```python
from build123d import *

# Parameters (mm, degrees)
SCHIZZO1_W                   = 205
SCHIZZO1_H                   = 100
ESTRUSIONE_ESTRUSIONE1_DEPTH = 20
SCHIZZO2_W                   = 20
SCHIZZO2_H                   = 100
ESTRUSIONE_ESTRUSIONE2_DEPTH = 65
TAGLIO_ESTRUSIONE1_DEPTH     = 20
SCHIZZO4_R                   = 9
TAGLIO_ESTRUSIONE2_DEPTH     = 20
SCHIZZO5_W                   = 60
SCHIZZO5_H                   = 29
ESTRUSIONE_ESTRUSIONE3_DEPTH = 15
FORO_FILETTATO_M8_1_D        = 6.8


with BuildPart() as part:
    # Schizzo1 → Estrusione-Estrusione1 (new body)
    with BuildSketch(Plane.XY):
        Rectangle(SCHIZZO1_W, SCHIZZO1_H)
    extrude(amount=ESTRUSIONE_ESTRUSIONE1_DEPTH)

    # Schizzo2 → Estrusione-Estrusione2 (add)
    with BuildSketch(Plane.XY.offset(20)):
        with Locations((67.5, 0)):
            Rectangle(SCHIZZO2_W, SCHIZZO2_H)
    extrude(amount=ESTRUSIONE_ESTRUSIONE2_DEPTH)

    # Schizzo3 → Taglio-Estrusione1 (cut)
    with BuildSketch(Plane.ZY.offset(-57.5)):
        with BuildLine():
            Line((65, 50), (85, 50))
            Line((85, 50), (85, 30))
            ThreePointArc((85, 30), (79.142135624, 44.142135624), (65, 50))
        make_face()
        with BuildLine():
            Line((85, -30), (85, -50))
            Line((85, -50), (65, -50))
            ThreePointArc((65, -50), (79.142135624, -44.142135624), (85, -30))
        make_face()
    extrude(amount=-TAGLIO_ESTRUSIONE1_DEPTH, mode=Mode.SUBTRACT)

    # Schizzo4 → Taglio-Estrusione2 (cut)
    with BuildSketch(Plane.ZY.offset(-57.5)):
        with Locations((45, 0)):
            Circle(SCHIZZO4_R)
    extrude(amount=-TAGLIO_ESTRUSIONE2_DEPTH, mode=Mode.SUBTRACT)

    # Schizzo5 → Estrusione-Estrusione3 (add)
    with BuildSketch(Plane.XY.offset(20)):
        with Locations((27.5, -35.5)):
            Rectangle(SCHIZZO5_W, SCHIZZO5_H)
        with Locations((27.5, 35.5)):
            Rectangle(SCHIZZO5_W, SCHIZZO5_H)
    extrude(amount=ESTRUSIONE_ESTRUSIONE3_DEPTH)

    # Foro filettato M8-1 (through all)
    with Locations(Plane(origin=(-80, 17, 20), x_dir=(1, 0, 0), z_dir=(0, 0, 1))):
        with Locations((0, 0), (0, -34)):
            Hole(FORO_FILETTATO_M8_1_D / 2)


solid = part.part
```
The model under review builds one solid part; all positions refer to its coordinate system, in mm. A direction names the side the tool comes from. Round coordinates to 2 decimals unless told otherwise and drop trailing zeros. Loops run counter-clockwise (first coordinate to the right, second up) from the corner with the lowest first, then second, coordinate; pieces in that order, holes last. Notation, with made-up numbers: (54, -22.75) - (98, -22.75) arc R6 cw to (98, -12.75) - close; hole circle Ø4 at (75.25, 38). An arc over 180 degrees is marked (long way). Write each question's results on one line, items separated by ' | '. Start each with the question number.
Q1. Take a section at B-B on y = -17. Give the boundary of the cut face in (x, z), plus the area to 3 significant figures.
Q2. Take a section at A-A on z = 45. Give the boundary of the cut face in (x, y), plus the area to 3 significant figures.
Q3. Take a section at C-C on x = -80. Give the boundary of the cut face in (y, z).
Q4. Insertion check: P1, Ø2, axis at x = 4, y = 15.5, coming from the +Z side; P2, Ø14.5, axis at y = 0, z = 45, coming from the -X side; P3, Ø14.5, axis at x = 32.5, y = 30.5, coming from the +Z side; P4, Ø10, axis at y = 29.5, z = 28.5, coming from the +X side. Each pin has a flat end and moves straight along its axis. Give the tip position at first contact, or say it passes through.
Q5. Tool access review of faces 4 (the flat face through (27, -21, 27)), 5 (the flat face through (90, 1, 20)), 6 (the flat face through (-102.5, -1, 10)), 7 (the flat face through (27, 36, 35)): name each direction out of +Z, -Z, +X, -X, +Y, -Y from which nothing blocks a thin tool from reaching the whole face with its end or side.
Q6. Take a section at D-D on x = 75. Give the boundary of the cut face in (y, z), plus the area to 3 significant figures.
Q7. Draft analysis for pull direction X (two halves, no side actions). For faces 1 (the flat face through (27, -35, 35)), 2 (the flat face through (-2.5, 35, 27)), 3 (the cylindrical face through (-77.302, 14.931, 9.86)), state which applies: pulls with the +X half, pulls with the -X half, needs draft (parallel to the pull), parting line crosses it, or undercut.
Q8. Wall thickness on line 1 along Y through (x, z) = (-80, 15.75); line 2 along Z through (x, y) = (-67, -34); line 3 along X through (y, z) = (18.5, 34): over which ranges is each line inside the solid? List them lowest first. Write a range as [from, to].
Data:
1) outline: (-102.5, 0) - (-83.4, 0) - (-83.4, 20) - (-102.5, 20) - close; (-76.6, 0) - (102.5, 0) - (102.5, 20) - (77.5, 20) - (77.5, 85) - (57.5, 85) - (57.5, 20) - (-76.6, 20) - close | area: 5,260 mm²
2) outline: (57.5, -50) - (77.5, -50) - (77.5, -9) - (57.5, -9) - close; (57.5, 9) - (77.5, 9) - (77.5, 50) - (57.5, 50) - close | area: 1,640 mm²
3) outline: (-50, 0) - (-20.4, 0) - (-20.4, 20) - (-50, 20) - close; (-13.6, 0) - (13.6, 0) - (13.6, 20) - (-13.6, 20) - close; (20.4, 0) - (50, 0) - (50, 20) - (20.4, 20) - close
4) P1: stops at z = 20 | P2: passes through | P3: stops at z = 35 | P4: stops at x = 77.5
5) face 4: +Z, -X | face 5: +Z, +X, +Y, -Y | face 6: +Z, -Z, -X, +Y, -Y | face 7: +Z, -X, +Y, -Y
6) outline: (-50, 0) - (50, 0) - (50, 65) arc R20 ccw to (30, 85) - (-30, 85) arc R20 ccw to (-50, 65) - close; hole circle Ø18 at (0, 45) | area: 8,070 mm²
7) face 1: needs draft | face 2: pulls with the -X half | face 3: undercut
8) line 1: y = [-50, -20.4], [-13.6, 13.6], [20.4, 50] | line 2: z = [0, 20] | line 3: x = [57.5, 77.5]
